Autodesk Inventor part; units mm, degrees
ref_plane "YZ Plane" through (0, 0, 0) normal (1, 0, 0) x (0, 1, 0)
ref_plane "XZ Plane" through (0, 0, 0) normal (0, 1, 0) x (-1, 0, 0)
ref_plane "XY Plane" through (0, 0, 0) normal (0, 0, 1) x (1, 0, 0)
sketch "Sketch1" plane through (0, 0, 0) normal (0, 1, 0) x (-1, 0, 0)
  line L0 (0, 0) -> (0, 28.5) construction
  line L1 (0, 28.5) -> (5.5858, 28.5) construction
  line L2 (6.2929, 28.7929) -> (7.7071, 30.2071) construction
  line L3 (8.4142, 30.5) -> (17.0754, 30.5) construction
  line L4 (17.7825, 30.2071) -> (23.2071, 24.7825) construction
  line L5 (23.5, 24.0754) -> (23.5, 18.7821) construction
  line L6 (23.6576, 18.2432) -> (29.0924, 9.7464) construction
  line L7 (29.25, 9.2075) -> (29.25, 0) construction
  line L8 (29.25, 0) -> (0, 0) construction
  arc A0 (29.25, 9.2075) -> (29.0924, 9.7464) centre (28.25, 9.2075) ccw construction
  arc A1 (23.5, 18.7821) -> (23.6576, 18.2432) centre (24.5, 18.7821) ccw construction
  arc A2 (23.5, 24.0754) -> (23.2071, 24.7825) centre (22.5, 24.0754) ccw construction
  arc A3 (17.7825, 30.2071) -> (17.0754, 30.5) centre (17.0754, 29.5) ccw construction
  arc A4 (8.4142, 30.5) -> (7.7071, 30.2071) centre (8.4142, 29.5) ccw construction
  arc A5 (5.5858, 28.5) -> (6.2929, 28.7929) centre (5.5858, 29.5) ccw construction
  line L9 (0, 28.5) -> (-5.5858, 28.5) construction
  line L10 (-6.2929, 28.7929) -> (-7.7071, 30.2071) construction
  line L11 (-8.4142, 30.5) -> (-17.0754, 30.5) construction
  line L12 (-17.7825, 30.2071) -> (-23.2071, 24.7825) construction
  line L13 (-23.5, 24.0754) -> (-23.5, 18.7821) construction
  line L14 (-23.6576, 18.2432) -> (-29.0924, 9.7464) construction
  line L15 (-29.25, 9.2075) -> (-29.25, 0) construction
  arc A6 (-29.0924, 9.7464) -> (-29.25, 9.2075) centre (-28.25, 9.2075) ccw construction
  arc A7 (-23.6576, 18.2432) -> (-23.5, 18.7821) centre (-24.5, 18.7821) ccw construction
  arc A8 (-23.2071, 24.7825) -> (-23.5, 24.0754) centre (-22.5, 24.0754) ccw construction
  arc A9 (-17.0754, 30.5) -> (-17.7825, 30.2071) centre (-17.0754, 29.5) ccw construction
  arc A10 (-7.7071, 30.2071) -> (-8.4142, 30.5) centre (-8.4142, 29.5) ccw construction
  arc A11 (-6.2929, 28.7929) -> (-5.5858, 28.5) centre (-5.5858, 29.5) ccw construction
  line L16 (0, -28.5) -> (5.5858, -28.5) construction
  line L17 (6.2929, -28.7929) -> (7.7071, -30.2071) construction
  line L18 (8.4142, -30.5) -> (17.0754, -30.5) construction
  line L19 (17.7825, -30.2071) -> (23.2071, -24.7825) construction
  line L20 (23.5, -24.0754) -> (23.5, -18.7821) construction
  line L21 (23.6576, -18.2432) -> (29.0924, -9.7464) construction
  line L22 (29.25, -9.2075) -> (29.25, 0) construction
  arc A12 (29.0924, -9.7464) -> (29.25, -9.2075) centre (28.25, -9.2075) ccw construction
  arc A13 (23.6576, -18.2432) -> (23.5, -18.7821) centre (24.5, -18.7821) ccw construction
  arc A14 (23.2071, -24.7825) -> (23.5, -24.0754) centre (22.5, -24.0754) ccw construction
  arc A15 (17.0754, -30.5) -> (17.7825, -30.2071) centre (17.0754, -29.5) ccw construction
  arc A16 (7.7071, -30.2071) -> (8.4142, -30.5) centre (8.4142, -29.5) ccw construction
  arc A17 (6.2929, -28.7929) -> (5.5858, -28.5) centre (5.5858, -29.5) ccw construction
  arc A18 (-23.5, -18.7821) -> (-23.6576, -18.2432) centre (-24.5, -18.7821) ccw construction
  line L23 (-23.6576, -18.2432) -> (-29.0924, -9.7464) construction
  arc A19 (-29.25, -9.2075) -> (-29.0924, -9.7464) centre (-28.25, -9.2075) ccw construction
  line L24 (-29.25, -9.2075) -> (-29.25, 0) construction
  line L25 (0, -28.5) -> (-5.5858, -28.5) construction
  line L26 (-6.2929, -28.7929) -> (-7.7071, -30.2071) construction
  line L27 (-8.4142, -30.5) -> (-17.0754, -30.5) construction
  line L28 (-23.5, -24.0754) -> (-23.5, -18.7821) construction
  arc A20 (-23.5, -24.0754) -> (-23.2071, -24.7825) centre (-22.5, -24.0754) ccw construction
  line L29 (-17.7825, -30.2071) -> (-23.2071, -24.7825) construction
  arc A21 (-17.7825, -30.2071) -> (-17.0754, -30.5) centre (-17.0754, -29.5) ccw construction
  arc A22 (-5.5858, -28.5) -> (-6.2929, -28.7929) centre (-5.5858, -29.5) ccw construction
  arc A23 (-8.4142, -30.5) -> (-7.7071, -30.2071) centre (-8.4142, -29.5) ccw construction
  line L30 (5.5858, -28) -> (0, -28)
  line L31 (0, -28) -> (-5.5858, -28)
  arc A24 (-5.5858, -28) -> (-6.6464, -28.4393) centre (-5.5858, -29.5) ccw
  line L32 (-6.6464, -28.4393) -> (-8.2071, -30)
  line L33 (-8.2071, -30) -> (-17.2825, -30)
  line L34 (-17.2825, -30) -> (-23, -24.2825)
  line L35 (-23, -24.2825) -> (-23, -18.7821)
  arc A25 (-23, -18.7821) -> (-23.2364, -17.9738) centre (-24.5, -18.7821) ccw
  line L36 (-23.2364, -17.9738) -> (-28.75, -9.3538)
  line L37 (-28.75, -9.3538) -> (-28.75, 0)
  line L38 (-28.75, 0) -> (-28.75, 9.3538)
  line L39 (-28.75, 9.3538) -> (-23.2364, 17.9738)
  arc A26 (-23.2364, 17.9738) -> (-23, 18.7821) centre (-24.5, 18.7821) ccw
  line L40 (-23, 18.7821) -> (-23, 24.2825)
  line L41 (-23, 24.2825) -> (-17.2825, 30)
  line L42 (-17.2825, 30) -> (-8.2071, 30)
  line L43 (-8.2071, 30) -> (-6.6464, 28.4393)
  arc A27 (-6.6464, 28.4393) -> (-5.5858, 28) centre (-5.5858, 29.5) ccw
  line L44 (-5.5858, 28) -> (0, 28)
  line L45 (0, 28) -> (5.5858, 28)
  arc A28 (5.5858, 28) -> (6.6464, 28.4393) centre (5.5858, 29.5) ccw
  line L46 (6.6464, 28.4393) -> (8.2071, 30)
  line L47 (8.2071, 30) -> (17.2825, 30)
  line L48 (17.2825, 30) -> (23, 24.2825)
  line L49 (23, 24.2825) -> (23, 18.7821)
  arc A29 (23, 18.7821) -> (23.2364, 17.9738) centre (24.5, 18.7821) ccw
  line L50 (23.2364, 17.9738) -> (28.75, 9.3538)
  line L51 (28.75, 9.3538) -> (28.75, 0)
  line L52 (28.75, 0) -> (28.75, -9.3538)
  line L53 (28.75, -9.3538) -> (23.2364, -17.9738)
  arc A30 (23.2364, -17.9738) -> (23, -18.7821) centre (24.5, -18.7821) ccw
  line L54 (23, -18.7821) -> (23, -24.2825)
  line L55 (23, -24.2825) -> (17.2825, -30)
  line L56 (17.2825, -30) -> (8.2071, -30)
  line L57 (8.2071, -30) -> (6.6464, -28.4393)
  arc A31 (6.6464, -28.4393) -> (5.5858, -28) centre (5.5858, -29.5) ccw
  line L58 (-50, 50) -> (50, 50)
  line L59 (50, 50) -> (50, -50)
  line L60 (50, -50) -> (-50, -50)
  line L61 (-50, -50) -> (-50, 50)
  line L62 (50, 0) -> (-50, 0) construction
  point P0 (6, 28.5)
  point P1 (17.4896, 30.5)
  point P2 (23.5, 24.4896)
  point P3 (23.5, 18.4896)
  point P4 (29.25, 9.5)
  point P5 (-6, 28.5)
  point P6 (-17.4896, 30.5)
  point P7 (-23.5, 24.4896)
  point P8 (-23.5, 18.4896)
  point P9 (-29.25, 9.5)
  point P10 (6, -28.5)
  point P11 (17.4896, -30.5)
  point P12 (23.5, -24.4896)
  point P13 (23.5, -18.4896)
  point P14 (29.25, -9.5)
  point P15 (-23.5, -18.4896)
  point P16 (-29.25, -9.5)
  point P17 (-6, -28.5)
  point P18 (-17.4896, -30.5)
  point P19 (-23.5, -24.4896)
  dimension "d0" = 45
  dimension "d1" = 6
  dimension "d2" = 30.5
  dimension "d3" = 28.5
  dimension "d4" = 29.25
  dimension "d5" = 6
  dimension "d6" = 9.5
  dimension "d7" = 23.5
  dimension "d8" = 8.5
  dimension "d9" = 1
  dimension "d10" = 0.5
  dimension "d11" = 100
extrude "Extrusion1" add sketch "Sketch1" along normal mid plane 1.6
equation "\"d10\" = offset"
equation "\"offset\" = 0.5"
properties part number "tarot_PCB_center"
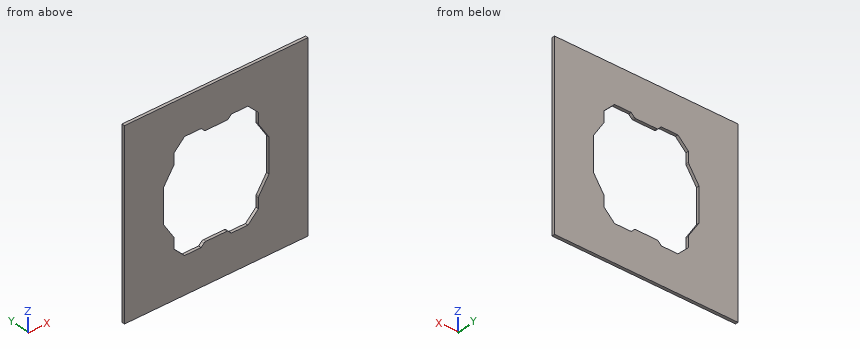
CAD build for the part. Positions are in the model's coordinates, mm. Round coordinates to 2 decimals unless told otherwise and drop trailing zeros. Order: outer loops, then holes, each group sorted by start corner. A loop starts at its lowest first (then second) coordinate and runs counter-clockwise, first axis right, second up.
Item 1: Saw through at B-B on x = 10. Write the cut outline in (y, z).
Item 2: Probe line 1 along Z through (x, y) = (11.5, -0.15); line 2 along Z through (x, y) = (5.5, -0.65); line 3 along X through (y, z) = (0.4, -5.5). List the from-to ranges inside material, lowest first.
Item 3: Saw through at A-A on z = 7. Write the cut outline in (x, y), then the cut area to 3 significant figures.
Reported:
1. outline: (-0.8, -50) - (0.8, -50) - (0.8, -30) - (-0.8, -30) - close; (-0.8, 30) - (0.8, 30) - (0.8, 50) - (-0.8, 50) - close
2. line 1: z = -50 to -30, 30 to 50
2. line 2: z = -50 to -28, 28 to 50
2. line 3: x = -50 to -28.75, 28.75 to 50
3. outline: (-50, -0.8) - (-28.75, -0.8) - (-28.75, 0.8) - (-50, 0.8) - close; (28.75, -0.8) - (50, -0.8) - (50, 0.8) - (28.75, 0.8) - close
3. area: 68.0 mm2
